The listing builds one solid part. Answer for the finished solid, in the listing's coordinates (mm). A direction names the side the tool comes from. Coordinates: 2 decimals unless noted, no trailing zeros. Order: outer loops, then holes, each group sorted by start corner. A loop starts at its lowest first (then second) coordinate and runs counter-clockwise, first axis right, second up. Notation, with made-up numbers: (12, 77) -> (25, 77) arc R16 cw to (25, 103) -> close; hole circle Ø1 at (46, 19.5). An arc over 180 degrees is marked (long way). Answer in a Markdown table with one row per item.
```python
from build123d import *
from OCP.BRepFilletAPI import BRepFilletAPI_MakeChamfer

# Parameters (mm, degrees)
CHAMFER1_SIZE  = 1
CHAMFER1_SIZE2 = 0.707106781


with BuildPart() as part:
    # Sketch1 → Revolve1 (revolve)
    with BuildSketch(Plane(origin=(0, 0, 0), x_dir=(1, 0, 0), z_dir=(0, 1, 0))):
        Polygon((59, 0), (54, 5), (54, 10), (59, 15), (4, 15), (4, 0), align=None)
    revolve(axis=Axis((0, 0, 0), (0, 0, -1)))

    # Chamfer1: one chamfer whose edges measure the first distance from different faces: ONE call of the kernel's chamfer builder (chamfer() names one face for all edges)
    chamfer1_edges_1 = [part.edges().sort_by_distance(p)[0] for p in [
        (-4, 0, 0),
        (-4, 0, -15),
    ]]
    chamfer1_edges_2 = [part.edges().sort_by_distance(p)[0] for p in [
        (-59, 0, 0),
    ]]
    chamfer1_side_2 = [part.faces().sort_by_distance(p)[0] for p in [
        (-56.5, 0, -2.5),
    ]]
    chamfer1_edges_3 = [part.edges().sort_by_distance(p)[0] for p in [
        (-59, 0, -15),
    ]]
    chamfer1_side_3 = [part.faces().sort_by_distance(p)[0] for p in [
        (-57.331227996, 0, -15),
    ]]
    chamfer1 = BRepFilletAPI_MakeChamfer(part.part.solid().wrapped)
    for e in chamfer1_edges_1:
        chamfer1.Add(CHAMFER1_SIZE, e.wrapped)
    for e in chamfer1_edges_2:
        chamfer1.Add(CHAMFER1_SIZE, CHAMFER1_SIZE2, e.wrapped, chamfer1_side_2[0].wrapped)  # the first distance lies on this face
    for e in chamfer1_edges_3:
        chamfer1.Add(CHAMFER1_SIZE, CHAMFER1_SIZE2, e.wrapped, chamfer1_side_3[0].wrapped)  # the first distance lies on this face
    add(Compound.cast(chamfer1.Shape()), mode=Mode.REPLACE)


solid = part.part
```
(1) Flat-ended cylindrical pins translate along their axes: pin 1 (12 mm diameter, centred on x = -4.5, y = 0, fed in from +Z); pin 2 (3 mm diameter, centred on y = -33.5, z = -8, fed in from +X); pin 3 (6 mm diameter, centred on x = 8, z = -4.5, fed in from -Y); pin 4 (8 mm diameter, centred on x = -28.5, z = -3, fed in from -Y). Find the tip coordinate at first contact, or state that the pin passes through.
Check values:
| item | result |
|---|---|
| pin 1 | z = 0 |
| pin 2 | x = 43.5 |
| pin 3 | y = -56.97 |
| pin 4 | y = -52.55 |
(2) A cutting plane is placed at A-A, the plane z = -12. Determine the outline of the cut face in (x, y).
Check values:
| item | result |
|---|---|
| outline | circle Ø112 at (0, 0); hole circle Ø8 at (0, 0) |
(3) For a pull along X with two mould halves and no side action, classify faces 4 (the flat face through (-12, -1, 0)), 5 (the cylindrical face through (-11.706, 52.716, -7.535)), 6 (the cylindrical face through (-0.867, 3.905, -7.409)) as released by +X, released by -X, zero draft, split by the parting line, or undercut.
Check values:
| item | result |
|---|---|
| face 4 | zero draft |
| face 5 | split by the parting line |
| face 6 | undercut |
(4) Which of the six approach directions +Z, -Z, +X, -X, +Y, -Y give full straight-line access (tool end or side, diameter ignored) to faces 1 (the conical face through (-11.8, 53, -10.3)), 2 (the conical face through (55.6, -17.51, -0.35)), 3 (the flat face through (-1, 12, -15))?
Check values:
| item | result |
|---|---|
| face 1 | none |
| face 2 | +Z |
| face 3 | -Z, +X, -X, +Y, -Y |
(5) Find the intervals of material crossed by line 1 along X through (y, z) = (0, -6); line 2 along Y through (x, z) = (0, -11.5), in increasing order. Write a range as from..to.
Check values:
| item | result |
|---|---|
| line 1 | -54..-4, 4..54 |
| line 2 | -55.5..-4, 4..55.5 |
